Answer from the drawing. Dimensions are ordinates in mm from the lowest x, y and z of the part. Coordinates: 2 decimals unless noted, no trailing zeros. Order: outer loops, then holes, each group sorted by start corner. A loop starts at its lowest first (then second) coordinate and runs counter-clockwise, first axis right, second up. Notation, with made-up numbers: (85.5, -34.75) -> (121.5, -34.75) arc R14 cw to (121.5, -29.75) -> close; hole circle Ø3 at (-11, 87). An arc over 180 degrees is marked (long way). Use CSV: the item, a comma, the result in double quotes.
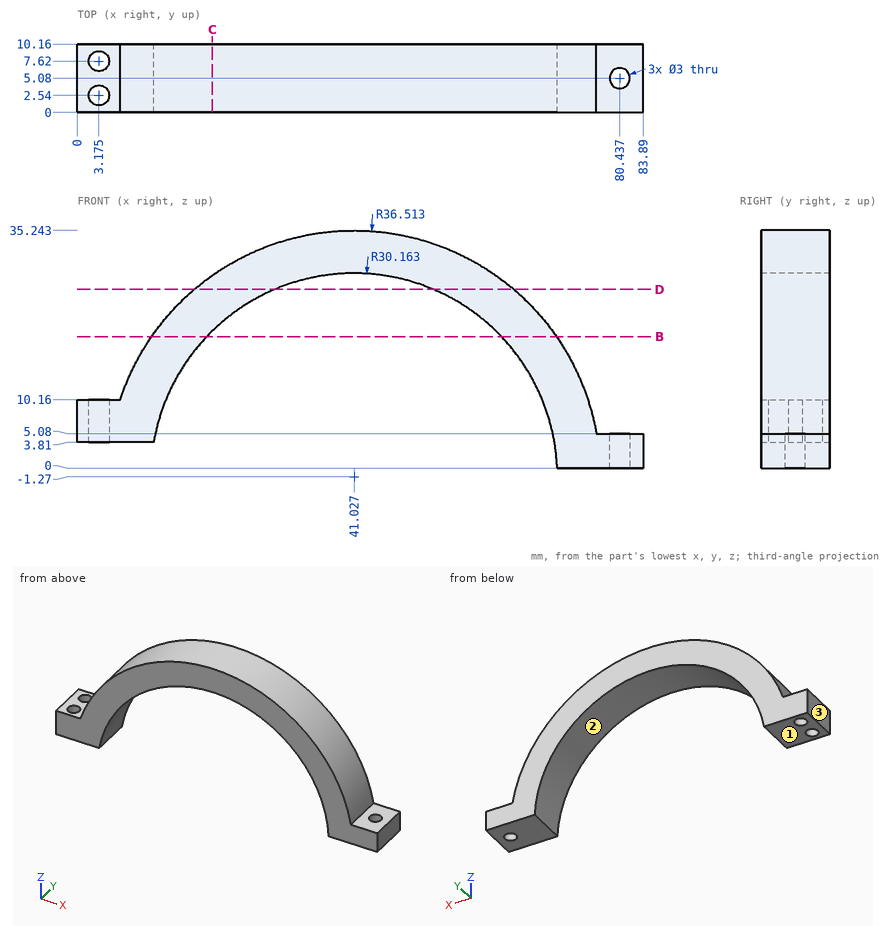
Item 1: Find section D-D, the plane z = 26.5. Give the vertices of the cut face in (x, y) (1 decimal).
Return value:
outline,"(17.3, 0) -> (29.3, 0) -> (29.3, 10.2) -> (17.3, 10.2) -> close; (52.8, 0) -> (64.7, 0) -> (64.7, 10.2) -> (52.8, 10.2) -> close"
Item 2: Find section B-B, the plane z = 19.5. Give the vertices of the cut face in (x, y) (1 decimal), then the cut area to 3 significant figures.
Return value:
outline,"(11, 0) -> (19.2, 0) -> (19.2, 10.2) -> (11, 10.2) -> close; (62.9, 0) -> (71.1, 0) -> (71.1, 10.2) -> (62.9, 10.2) -> close"
area,"166 mm^2"
Item 3: Find section C-C, the plane x = 20. Give the vertices of the cut face in (y, z) (1 decimal).
Return value:
outline,"(0, 20.4) -> (10.2, 20.4) -> (10.2, 28.6) -> (0, 28.6) -> close"
Item 4: Each of these flat-tipped pins is pushed along its axis until it touches: P1, Ø1.9, axis at x = 2.5, y = 4, coming from the +Z side; P2, Ø1, axis at x = 57.5, y = 6, coming from the +Z side; P3, Ø3.5, axis at x = 3.175, y = 2.54, coming from the -Z side. Where does it stop, or does it pass through?
Return value:
P1,"stops at z = 10.16"
P2,"stops at z = 31.56"
P3,"stops at z = 3.81"
Item 5: Straight lines are drawn through the part: line 1 along X through (y, z) = (4.25, 4.5) (1 decimal); line 2 along X through (y, z) = (6.5, 8) (1 decimal); line 3 along Z through (x, y) = (5.5, 7). For each, find the intervals that lie inside material, in ascending order.
Return value:
line 1,"x = 0 to 11.4, 70.6 to 79.2, 81.7 to 83.9"
line 2,"x = 0 to 2.2, 4.2 to 12.3, 69.7 to 76.3"
line 3,"z = 3.81 to 10.16"
Item 6: The mould has two halves that part along X. Classify the marked faces 1, 2 and 3: +X half, -X half, draft (parallel to the pull), parting line (faces both ways), or undercut.
Return value:
face 1,"draft"
face 2,"undercut"
face 3,"-X half"
